Drawing for the job (mm, zero at the part's lowest x, y, z). A direction names the side the tool comes from. Give positions to 0.01 mm unless a question says otherwise; leave off trailing zeros. Loops run counter-clockwise (first coordinate to the right, second up) from the corner with the lowest first, then second, coordinate; pieces in that order, holes last. Notation, with made-up numbers: (-2, -7) -> (36, -7) arc R26 ccw to (36, 32) -> close; hole circle Ø3 at (5, -30). An arc over 180 degrees is marked (long way). Use CSV: the item, a comma, the result in double quotes. Start each with the question number.
(1) Cut at C-C on y = 7. Write the cut outline in (x, z), then the cut area to 3 significant figures.
(2) Flat gauge pins, fed straight in: pin 1 (0.8 mm diameter, centred on x = 7.5, y = 9.5, fed in from -Z); pin 2 (0.5 mm diameter, centred on y = 9.5, z = 9, fed in from -X). Where does each tip first touch, or does it go through?
(3) 3-axis set-ups, long thin cutter, end or side, ignore diameter. For the marked faces 1 and 2: which of +Z, -Z, +X, -X, +Y, -Y reach the whole face in a straight line?
(4) Cut at D-D on y = 9.25. Write the cut outline in (x, z), then the cut area to 3 significant figures.
(5) Cut at B-B on z = 17.75. Write the cut outline in (x, y), then the cut area to 3 significant figures.
(6) Drill centre lines: probe 1 along X at (y, z) = (5.5, 4.25); probe 2 along Z at (x, y) = (9, 9.5). Where is each one in solid material? Low to high.
(7) Pull direction Y, two halves, no side cores. Call the marked faces 3, 4, 5 and 6: pulls with the +Y half, pulls with the -Y half, needs draft (parallel to the pull), parting line crosses it, or undercut.
(8) Cut at A-A on x = 3.25. Write the cut outline in (y, z).
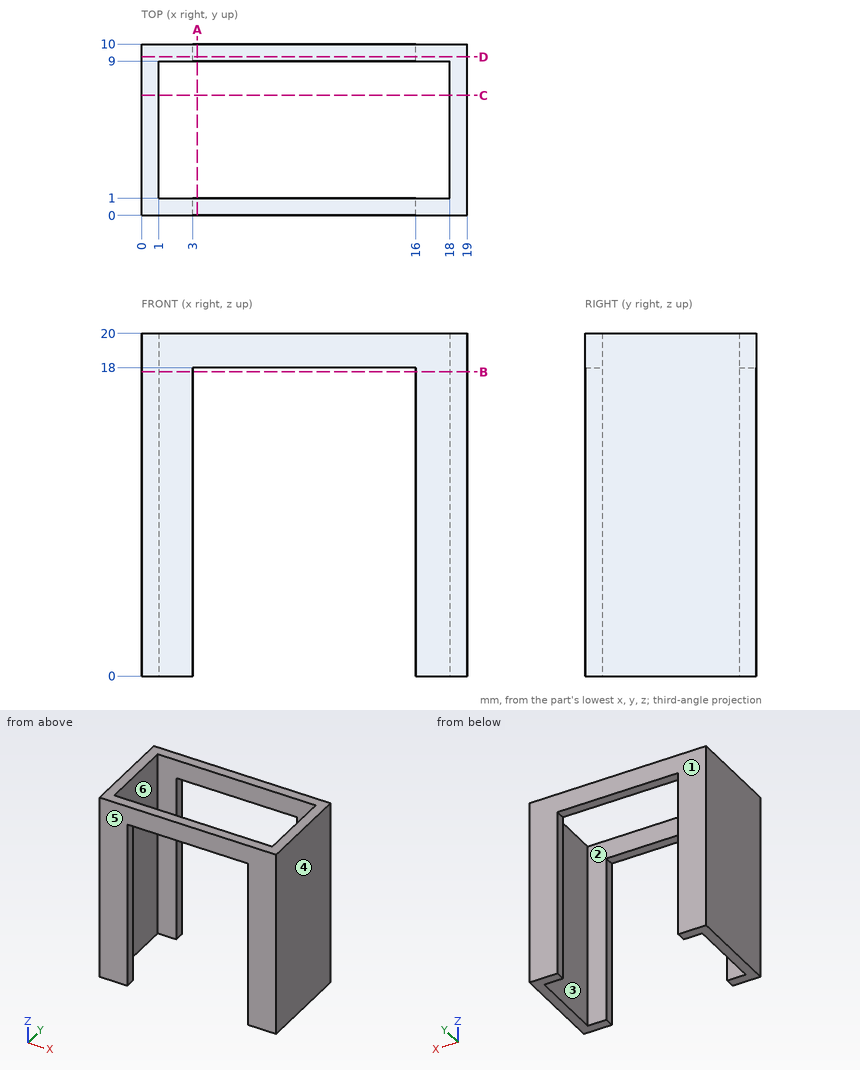
Check result:
1,outline,"(0, 0) -> (1, 0) -> (1, 20) -> (0, 20) -> close; (18, 0) -> (19, 0) -> (19, 20) -> (18, 20) -> close"
1,area,"40.0 mm²"
2,pin 1,"z = 18"
2,pin 2,"x = 0"
3,face 1,"+Z, -Z, +X, -X, +Y"
3,face 2,"+Z, -Z"
4,outline,"(0, 0) -> (3, 0) -> (3, 18) -> (16, 18) -> (16, 0) -> (19, 0) -> (19, 20) -> (0, 20) -> close"
4,area,"146 mm²"
5,outline,"(0, 0) -> (3, 0) -> (3, 1) -> (1, 1) -> (1, 9) -> (3, 9) -> (3, 10) -> (0, 10) -> close; (16, 0) -> (19, 0) -> (19, 10) -> (16, 10) -> (16, 9) -> (18, 9) -> (18, 1) -> (16, 1) -> close"
5,area,"28.0 mm²"
6,probe 1,"0 to 1, 18 to 19"
6,probe 2,"18 to 20"
7,face 3,"undercut"
7,face 4,"needs draft"
7,face 5,"pulls with the -Y half"
7,face 6,"undercut"
8,outline,"(0, 18) -> (1, 18) -> (1, 20) -> (0, 20) -> close; (9, 18) -> (10, 18) -> (10, 20) -> (9, 20) -> close"
